Design review of the part built by this model. Coordinates are the model's own, in mm. Face numbers are marked on the shaded views. A direction names the side the tool comes from. Give positions to 0.01 mm unless a question says otherwise; leave off trailing zeros. Loops run counter-clockwise (first coordinate to the right, second up) from the corner with the lowest first, then second, coordinate; pieces in that order, holes last. Notation, with made-up numbers: (-38.75, 1) -> (-17.75, 1) arc R25 cw to (-17.75, 38) -> close; hole circle Ø10 at (-31, 61.25). An arc over 180 degrees is marked (long way). Answer in a Markdown table with one row per item. Add a question column.
(1) Consider section D-D on x = -121. Write out the cut boundary in (y, z) (3 decimals), then the cut area to 3 significant figures.
(2) For line 1 (Y direction, x = -101.6, z = 6.25); line 2 (X direction, y = 14, z = 7.5); line 3 (X direction, y = -12, z = 5), list the stretches that pass through material, from the lowest coordinate up.
(3) For the marked faces 1, 2 and 3, list the 3-axis set-ups (+Z, -Z, +X, -X, +Y, -Y) from which the entire face can be reached by the end or side of a thin tool; tool diameter is ignored.
(4) Consider section B-B on y = 0. Count the separate pieces of the cut face and the enclosed holes in it, then the cut area to 3 significant figures.
(5) Consider section C-C on y = 12.7. Write out the cut boundary in (x, z) (3 decimals), then the cut area to 3 significant figures.
(6) Consider section A-A on x = -31.75. Write out the cut boundary in (y, z) (3 decimals), then the cut area to 3 significant figures.
(7) For pin 1 (4 mm diameter, centred on y = -7, z = 3.5, fed in from -X); pin 2 (1 mm diameter, centred on x = -23, z = 7, fed in from -Y) (3 decimals); pin 3 (4 mm diameter, centred on y = 12, z = 3.5, fed in from -X), all flat-tipped, find the tip position at first contact; note any pin that passes through.
(8) Draft analysis for pull direction X (two halves, no side actions). For the marked faces 4, 5, 6 and 7, state which applies: +X half, -X half, draft (parallel to the pull), parting line (faces both ways), or undercut.
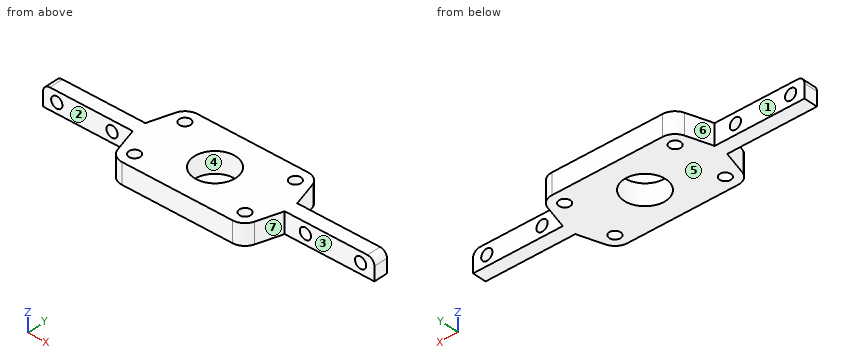
Autodesk Inventor part; units mm, degrees
ref_plane "YZ Plane" through (0, 0, 0) normal (1, 0, 0) x (0, 1, 0)
ref_plane "XZ Plane" through (0, 0, 0) normal (0, 1, 0) x (-1, 0, 0)
ref_plane "XY Plane" through (0, 0, 0) normal (0, 0, 1) x (1, 0, 0)
sketch "Sketch1" plane through (0, 0, 0) normal (0, 1, 0) x (-1, 0, 0)
  line L0 (0, 0) -> (152.4, 0)
  line L1 (152.4, 0) -> (152.4, 6.35)
  line L2 (34.925, 9.525) -> (3.175, 9.525)
  line L3 (0, 6.35) -> (0, 0)
  circle A0 centre (6.35, 4.7625) radius 2.5797
  circle A1 centre (31.75, 4.7625) radius 2.5797
  circle A2 centre (120.65, 4.7625) radius 2.5797
  circle A3 centre (146.05, 4.7625) radius 2.5797
  line L4 (38.1, 9.525) -> (114.3, 9.525)
  line L5 (114.3, 6.35) -> (114.3, 4.7625)
  line L6 (38.1, 4.7625) -> (38.1, 6.35)
  arc A4 (38.1, 6.35) -> (34.925, 9.525) centre (34.925, 6.35) ccw
  arc A5 (3.175, 9.525) -> (0, 6.35) centre (3.175, 6.35) ccw
  line L7 (117.475, 9.525) -> (149.225, 9.525)
  arc A6 (117.475, 9.525) -> (114.3, 6.35) centre (117.475, 6.35) ccw
  arc A7 (152.4, 6.35) -> (149.225, 9.525) centre (149.225, 6.35) ccw
  line L8 (114.3, 6.35) -> (114.3, 0)
  line L9 (38.1, 6.35) -> (38.1, 0)
  line L10 (114.3, 4.7625) -> (114.3, 9.525)
  line L11 (117.475, 9.525) -> (114.3, 9.525)
  line L12 (38.1, 6.35) -> (38.1, 9.525)
  line L13 (38.1, 9.525) -> (34.925, 9.525)
  line L14 (38.1, 3.175) -> (114.3, 3.175)
  line L15 (88.9, 3.175) -> (116.778, 9.4476)
  line L16 (63.5, 3.175) -> (35.622, 9.4476)
  point P0 (152.4, 9.525)
  point P1 (0, 9.525)
  point P2 (114.3, 3.175)
  dimension "d0" = 152.4
  dimension "d1" = 9.525
  dimension "d2" = 4.7625
  dimension "d3" = 4.7625
  dimension "d4" = 4.7625
  dimension "d5" = 4.7625
  dimension "d6" = 25.4
  dimension "d7" = 25.4
  dimension "d8" = 5.1594
  dimension "d9" = 6.35
  dimension "d10" = 6.35
  dimension "d11" = 4.7625
  dimension "d12" = 6.35
  dimension "d13" = 6.35
  dimension "d14" = 3.175
  dimension "d15" = 3.175
  dimension "d37" = 3.175
  dimension "d100" = 25.4
extrude "Extrusion1" add sketch "Sketch1" along normal mid plane 6.35
extrude "Extrusion2" add sketch "Sketch1" along normal mid plane 50.8 contours L9 L14 L8 L0 | L9 L6 L12 L16 L14 | L14 L15 L10 L5 L8 | L16 L12 L4 L10 L15 L14
sketch "Sketch4" plane through (-38.1, 25.4, 0) normal (0, 0, -1) x (-1, 0, 0)
  line L0 (76.2, -50.8) -> (76.2, -28.575)
  line L1 (0, 0) -> (76.2, 0)
  line L2 (76.2, 0) -> (76.2, -50.8)
  line L3 (76.2, -50.8) -> (0, -50.8)
  line L4 (0, -50.8) -> (0, 0)
  circle A0 centre (38.1, -25.4) radius 9.525
  circle A1 centre (12.7, -12.7) radius 2.5797
  circle A2 centre (12.7, -38.1) radius 2.5797
  circle A3 centre (63.5, -12.7) radius 2.5797
  circle A4 centre (63.5, -38.1) radius 2.5797
  circle A5 centre (12.7, -12.7) radius 6.35
  circle A6 centre (12.7, -38.1) radius 6.35
  circle A7 centre (63.5, -12.7) radius 6.35
  circle A8 centre (63.5, -38.1) radius 6.35
  line L5 (12.7, -6.35) -> (63.5, -6.35)
  line L6 (69.85, -11.1925) -> (69.85, -39.6075)
  line L7 (63.5, -44.45) -> (12.7, -44.45)
  line L8 (6.35, -39.6075) -> (6.35, -11.1925)
  line L9 (-38.1, -22.225) -> (6.35, -22.225)
  line L10 (6.35, -22.225) -> (6.35, -28.575)
  line L11 (6.35, -28.575) -> (-38.1, -28.575)
  line L12 (-38.1, -28.575) -> (-38.1, -22.225)
  line L13 (69.85, -22.225) -> (114.3, -22.225)
  line L14 (114.3, -22.225) -> (114.3, -28.575)
  line L15 (114.3, -28.575) -> (69.85, -28.575)
  line L16 (69.85, -28.575) -> (69.85, -22.225)
  line L17 (-38.1, -28.575) -> (-38.1, -22.225)
  line L18 (0, -28.575) -> (-38.1, -28.575)
  line L19 (3.175, -22.225) -> (6.6234, -10.8567)
  line L20 (3.175, -28.575) -> (6.6234, -39.9433)
  line L21 (69.5766, -10.8567) -> (73.025, -22.225)
  line L22 (73.025, -28.575) -> (69.5766, -39.9433)
  point P0 (-38.1, -25.4)
  point P1 (-38.1, -25.4)
  point P2 (7.0276, -9.8458)
  point P3 (0, -22.225)
  point P4 (7.0276, -40.9542)
  point P5 (76.2, -22.225)
  point P6 (69.1724, -9.8458)
  point P7 (69.1724, -40.9542)
  point P8 (0, -22.225)
  dimension "d71" = 76.2
  dimension "d72" = 50.8
  dimension "d73" = 25.4
  dimension "d74" = 38.1
  dimension "d75" = 19.05
  dimension "d78" = 25.4
  dimension "d81" = 50.8
  dimension "d84" = 12.7
  dimension "d85" = 12.7
  dimension "d86" = 5.1594
  dimension "d87" = 12.7
  dimension "d90" = 25.4
  dimension "d93" = 50.8
  dimension "d96" = 3.175
  dimension "d97" = 6.35
  dimension "d111" = 3.175
extrude "Extrusion5" cut sketch "Sketch4" against normal through all contours L3 L4 L11 L20 A6 L7 A8 L22 L15 L0 | L13 L21 A7 L5 A5 L19 L9 L4 L1 L2 | A0 | A1 | A2 | A3 | A4
equation "\"d2\" = 0.5 * d1"
equation "\"d3\" = d2"
equation "\"d4\" = d2"
equation "\"d5\" = d2"
equation "\"d10\" = d9"
equation "\"d11\" = 0.5 * d1"
equation "\"d37\" = 0.333333 * d1"
properties part number "Face Plate"
Values follow:
| question | item | result |
|---|---|---|
| 1 | outline | (-3.175, 0) -> (3.175, 0) -> (3.175, 2.207) -> (-3.175, 2.207) -> close; (-3.175, 7.318) -> (3.175, 7.318) -> (3.175, 9.525) -> (-3.175, 9.525) -> close |
| 1 | area | 28.0 mm2 |
| 2 | line 1 | -19.05 to -15.28, -10.12 to 10.12, 15.28 to 19.05 |
| 2 | line 2 | -107.84 to -103.83, -99.37 to -53.03, -48.57 to -44.56 |
| 2 | line 3 | -108.45 to -104.08, -99.12 to -53.28, -48.32 to -43.95 |
| 3 | face 1 | +Z, -Z, -X, +Y |
| 3 | face 2 | +Z, -Z, -X, -Y |
| 3 | face 3 | +Z, -Z, +X, -Y |
| 4 | separate pieces | 2 |
| 4 | enclosed holes | 4 |
| 4 | area | 1,180 mm2 |
| 5 | outline | (-108.236, 0) -> (-104.18, 0) -> (-104.18, 9.525) -> (-108.236, 9.525) -> close; (-99.02, 0) -> (-53.38, 0) -> (-53.38, 9.525) -> (-99.02, 9.525) -> close; (-48.22, 0) -> (-44.164, 0) -> (-44.164, 9.525) -> (-48.22, 9.525) -> close |
| 5 | area | 512 mm2 |
| 6 | outline | (-3.175, 0) -> (3.175, 0) -> (3.175, 2.183) -> (-3.175, 2.183) -> close; (-3.175, 7.342) -> (3.175, 7.342) -> (3.175, 9.525) -> (-3.175, 9.525) -> close |
| 6 | area | 27.7 mm2 |
| 7 | pin 1 | x = -110.57 |
| 7 | pin 2 | y = -3.175 |
| 7 | pin 3 | x = -109.05 |
| 8 | face 4 | undercut |
| 8 | face 5 | draft |
| 8 | face 6 | -X half |
| 8 | face 7 | +X half |
